Part model, mm, in its own coordinate system. Face numbers are marked on the shaded views. Give positions to 0.01 mm unless a question says otherwise; leave off trailing zeros. Order: outer loops, then holes, each group sorted by start corner. A loop starts at its lowest first (then second) coordinate and runs counter-clockwise, first axis right, second up. Notation, with made-up numbers: (35, 67) - (73, 67) arc R14 ccw to (73, 72) - close; hole circle Ø7 at (69.5, 29). An arc over 180 degrees is marked (long way). Use one line per item in the form item = value. Start each with the question number.
1. Pin check, flat tips, straight feed: P1, Ø3, axis at x = 9, z = 3, coming from the -Y side; P2, Ø2, axis at x = -3.5, z = 3, coming from the +Y side. Stop position of each tip, or through.
2. Band-saw the part on D-D, the plane y = 2. List the corners of the cut face in (x, z).
3. Band-saw the part on A-A, the plane y = -1. List the corners of the cut face in (x, z).
4. Band-saw the part on B-B, the plane z = 3. List the corners of the cut face in (x, y), plus the area to 3 significant figures.
5. Pull direction X, two halves, no side cores. Call the marked faces 1, 2, 3 and 4: +X half, -X half, draft (parallel to the pull), parting line (faces both ways), or undercut.
6. Drill centre lines: line 1 (Y direction, x = 3.5, z = 3); line 2 (X direction, y = 2.75, z = 3); line 3 (X direction, y = 2, z = 3.5). Where is each one in solid material? Low to high.
7. Band-saw the part on C-C, the plane x = -9. List the corners of the cut face in (y, z), plus the area to 3 significant figures.
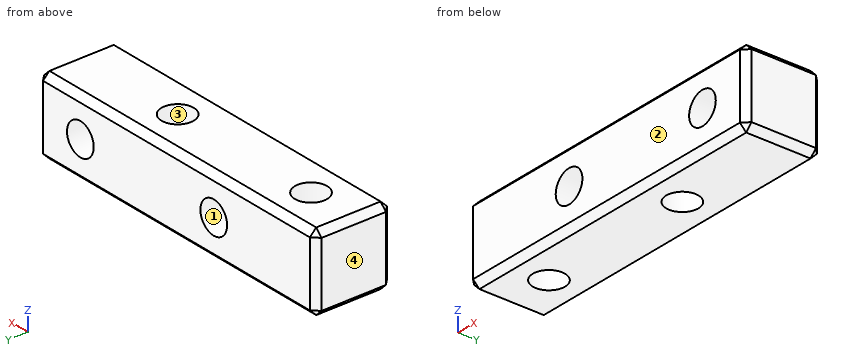
from build123d import *

# Parameters (mm, degrees)
SKETCH_1_W         = 26
SKETCH_1_H         = 6
EXTRUDE_1_DEPTH    = 6
CHAMFER_1_SIZE     = 0.5
HOLE_WIZARD_M3_1_D = 2.5
HOLE_WIZARD_M3_2_D = 2.5


with BuildPart() as part:
    # 草图1 → 凸台-拉伸1 (new body)
    with BuildSketch(Plane.XY):
        Rectangle(SKETCH_1_W, SKETCH_1_H)
    extrude(amount=EXTRUDE_1_DEPTH)

    # 倒角1
    chamfer_1_edges = [part.edges().sort_by_distance(p)[0] for p in [
        (-13, 0, 6),
        (0, -3, 6),
        (13, 0, 6),
        (0, -3, 0),
        (-13, 0, 0),
        (0, 3, 0),
        (13, 0, 0),
        (13, -3, 3),
        (-13, -3, 3),
        (-13, 3, 3),
        (13, 3, 3),
        (0, 3, 6),
    ]]
    chamfer(chamfer_1_edges, length=CHAMFER_1_SIZE)

    # M3 螺纹孔1 (through all)
    with Locations(Plane(origin=(-9, 0, 6), x_dir=(1, 0, 0), z_dir=(0, 0, 1))):
        with Locations((0, 0), (12.5, 0)):
            Hole(HOLE_WIZARD_M3_1_D / 2)

    # M3 螺纹孔2 (through all)
    with Locations(Plane(origin=(-3.5, 3, 3), x_dir=(0, 0, 1), z_dir=(0, 1, 0))):
        with Locations((0, 0), (0, 12.5)):
            Hole(HOLE_WIZARD_M3_2_D / 2)


solid = part.part
From the geometry:
q1.P1 = -3
q1.P2 = through
q2.outline = (-13, 0.5) - (-12.5, 0) - (12.5, 0) - (13, 0.5) - (13, 5.5) - (12.5, 6) - (-12.5, 6) - (-13, 5.5) - close; hole circle Ø2.5 at (-3.5, 3); hole circle Ø2.5 at (9, 3)
q3.outline = (-13, 0.5) - (-12.5, 0) - (-9.75, 0) - (-9.75, 6) - (-12.5, 6) - (-13, 5.5) - close; (-8.25, 0) - (2.75, 0) - (2.75, 6) - (-8.25, 6) - close; (4.25, 0) - (12.5, 0) - (13, 0.5) - (13, 5.5) - (12.5, 6) - (4.25, 6) - close; hole circle Ø2.5 at (-3.5, 3); hole circle Ø2.5 at (9, 3)
q4.outline = (-13, -2.5) - (-12.5, -3) - (-4.75, -3) - (-4.75, 3) - (-12.5, 3) - (-13, 2.5) - close; (-2.25, -3) - (7.75, -3) - (7.75, 3) - (-2.25, 3) - close; (10.25, -3) - (12.5, -3) - (13, -2.5) - (13, 2.5) - (12.5, 3) - (10.25, 3) - close; hole circle Ø2.5 at (-9, 0); hole circle Ø2.5 at (3.5, 0)
q4.area = 116 mm²
q5.face_1 = undercut
q5.face_2 = draft
q5.face_3 = undercut
q5.face_4 = -X half
q6.line_1 = -3 to -1.25, 1.25 to 3
q6.line_2 = -12.75 to -4.75, -2.25 to 7.75, 10.25 to 12.75
q6.line_3 = -13 to -4.65, -2.35 to 7.85, 10.15 to 13
q7.outline = (-3, 0.5) - (-2.5, 0) - (-1.25, 0) - (-1.25, 6) - (-2.5, 6) - (-3, 5.5) - close; (1.25, 0) - (2.5, 0) - (3, 0.5) - (3, 5.5) - (2.5, 6) - (1.25, 6) - close
q7.area = 20.5 mm²
